```python
from build123d import *

# Parameters (mm, degrees)
ESQUISSE1_R                  = 1.15
ESQUISSE1_R_2                = 13.5
BOSS_EXTRU_1_DEPTH           = 8
ESQUISSE2_R                  = 13.5
ESQUISSE2_R_2                = 12.5
BOSS_EXTRU_2_DEPTH           = 2
ENL_V_MAT_EXTRU_1_DEPTH      = 3
R_P_TITION_CIRCULAIRE1_COUNT = 3
ESQUISSE4_W                  = 10
ESQUISSE4_H                  = 20
BOSS_EXTRU_3_DEPTH           = 40
PER_AGEAVANC_1_OUTLINE_R     = 2.25
PER_AGEAVANC_1_DEPTH         = 2.45
PER_AGEAVANC_1_DRAFT         = 45
PER_AGEAVANC_1_2_OUTLINE_R   = 2.25
PER_AGEAVANC_1_2_DEPTH       = 2.45
PER_AGEAVANC_1_2_DRAFT       = 45
ESQUISSE7_R                  = 2.25
ENL_V_MAT_EXTRU_2_DEPTH      = 66.754160325
CHANFREIN1_SIZE              = 1


# Read off the part's stored shape, not the designer's step: PerçageAvancé1
with BuildPart() as part:
    # Esquisse1 → Boss.-Extru.1 (new body)
    with BuildSketch(Plane(origin=(0, 0, 0), x_dir=(1, 0, 0), z_dir=(0, 1, 0))):
        with BuildLine():
            Line((20, -46.91), (20, 0))
            ThreePointArc((20, 0), (0, 20), (-20, 0))
            Line((-20, 0), (-20, -46.91))
            Line((-20, -46.91), (20, -46.91))
        make_face()
        with Locations(Location((0, 16.5, 0), (0, 0, 270))):
            Circle(ESQUISSE1_R, mode=Mode.SUBTRACT)
        with Locations(Location((-14.289419162, -8.25, 0), (0, 0, 270))):
            Circle(ESQUISSE1_R, mode=Mode.SUBTRACT)
        with Locations(Location((0, 0, 0), (0, 0, 270))):
            Circle(ESQUISSE1_R_2, mode=Mode.SUBTRACT)
        with Locations(Location((14.289419162, -8.25, 0), (0, 0, 270))):
            Circle(ESQUISSE1_R, mode=Mode.SUBTRACT)
    extrude(amount=BOSS_EXTRU_1_DEPTH)

    # Esquisse2 → Boss.-Extru.2 (add)
    with BuildSketch(Plane.XZ):
        with Locations(Location((0, 0, 0), (0, 0, 270))):
            Circle(ESQUISSE2_R)
        with Locations(Location((0, 0, 0), (0, 0, 270))):
            Circle(ESQUISSE2_R_2, mode=Mode.SUBTRACT)
    extrude(amount=-BOSS_EXTRU_2_DEPTH)

    # Esquisse3 → Enlèv. mat.-Extru.1 (cut)
    with BuildSketch(Plane.XZ):
        Polygon((-14.289419162, 5.882863896), (-12.239419162, 7.066431948), (-12.239419162, 9.433568052), (-14.289419162, 10.617136104), (-16.339419162, 9.433568052), (-16.339419162, 7.066431948), align=None)
    enl_v_mat_extru_1 = extrude(amount=-ENL_V_MAT_EXTRU_1_DEPTH, mode=Mode.SUBTRACT)

    # Répétition circulaire1: Enlèv. mat.-Extru.1 ×3 about axis
    r_p_tition_circulaire1_axis = Axis((0, 0, 0), (0, 1, 0))
    for i in range(1, R_P_TITION_CIRCULAIRE1_COUNT):
        add(enl_v_mat_extru_1.rotate(r_p_tition_circulaire1_axis, i * 360 / R_P_TITION_CIRCULAIRE1_COUNT), mode=Mode.SUBTRACT)

    # Esquisse4 → Boss.-Extru.3 (add)
    with BuildSketch(Plane.ZY.offset(20)):
        with Locations((41.91, 10)):
            Rectangle(ESQUISSE4_W, ESQUISSE4_H)
    extrude(amount=-BOSS_EXTRU_3_DEPTH)


with BuildPart() as per_ageavanc_1_tool:
    # PerçageAvancé1 outline → PerçageAvancé1 (with draft: the straight prism first)
    with BuildSketch(Plane.XY.offset(39.36)):
        with Locations((-12, 14)):
            Circle(PER_AGEAVANC_1_OUTLINE_R)
    extrude(amount=-PER_AGEAVANC_1_DEPTH)
    # PerçageAvancé1: the draft: its side faces are tilted about the plane it starts from
    per_ageavanc_1_sides = [per_ageavanc_1_tool.faces().sort_by_distance(p)[0] for p in [
        (-14.25, 14, 38.135),
    ]]
    draft(per_ageavanc_1_sides, Plane.XY.offset(39.36), PER_AGEAVANC_1_DRAFT)


with BuildPart() as part_1:
    add(part.part)

    # PerçageAvancé1: cut by per_ageavanc_1_tool
    add(per_ageavanc_1_tool.part, mode=Mode.SUBTRACT)


with BuildPart() as per_ageavanc_1_2_tool:
    # Per_ageAvanc_1 2 outline → Per_ageAvanc_1 2 (with draft: the straight prism first)
    with BuildSketch(Plane.XY.offset(39.36)):
        with Locations((12, 14)):
            Circle(PER_AGEAVANC_1_2_OUTLINE_R)
    extrude(amount=-PER_AGEAVANC_1_2_DEPTH)
    # Per_ageAvanc_1 2: the draft: its side faces are tilted about the plane it starts from
    per_ageavanc_1_2_sides = [per_ageavanc_1_2_tool.faces().sort_by_distance(p)[0] for p in [
        (9.75, 14, 38.135),
    ]]
    draft(per_ageavanc_1_2_sides, Plane.XY.offset(39.36), PER_AGEAVANC_1_2_DRAFT)


with BuildPart() as part_2:
    add(part_1.part)

    # Per_ageAvanc_1 2: cut by per_ageavanc_1_2_tool
    add(per_ageavanc_1_2_tool.part, mode=Mode.SUBTRACT)

    # Esquisse7 → Enlèv. mat.-Extru.2 (cut, through all)
    with BuildSketch(Plane(origin=(0, 0, 39.36), x_dir=(-1, 0, 0), z_dir=(0, 0, -1))):
        with Locations((-12, 14)):
            Circle(ESQUISSE7_R)
        with Locations((12, 14)):
            Circle(ESQUISSE7_R)
    extrude(amount=-ENL_V_MAT_EXTRU_2_DEPTH, mode=Mode.SUBTRACT)

    # Chanfrein1
    chanfrein1_edges = [part_2.edges().sort_by_distance(p)[0] for p in [
        (20, 8, 18.455),
        (20, 14, 36.91),
        (0, 20, 36.91),
        (-20, 14, 36.91),
        (-20, 8, 18.455),
        (0, 8, -20),
        (0, 0, -20),
        (0, 8, -13.5),
        (20, 0, 23.455),
        (-20, 0, 23.455),
    ]]
    chamfer(chanfrein1_edges, length=CHANFREIN1_SIZE)


solid = part_2.part
```
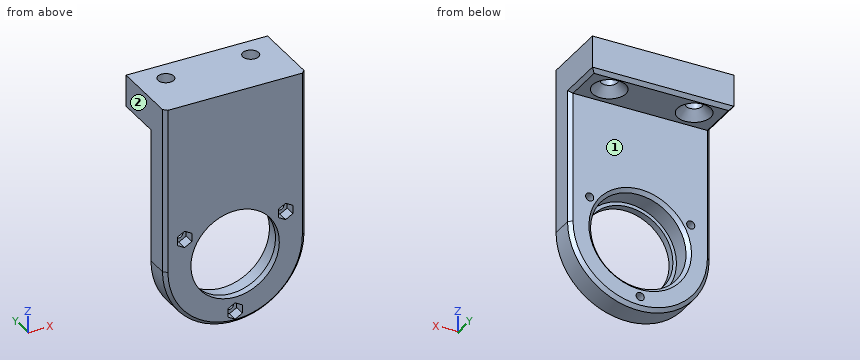
Could you check a few things on this model? Use its own coordinates, in mm. Face numbers are marked on the shaded views. A direction names the side the tool comes from. Round coordinates to 2 decimals unless told otherwise and drop trailing zeros. Loops run counter-clockwise (first coordinate to the right, second up) from the corner with the lowest first, then second, coordinate; pieces in that order, holes last. Notation, with made-up numbers: M 51,23.5 L 101,23.5 A21 cw 101,41.5 Z; hole C -39.75,28.25 d6. An arc over 180 degrees is marked long. Write item = value, one per line.
1. I want a section at A-A, the plane y = 5. Write out the boundary of the cut face in (x, z), and give its area (3 significant figures).
Results below:
outline = M -20,0 A20 ccw 20,0 L 20,46.91 L -20,46.91 Z; hole C -14.29,8.25 d2.3; hole C 0,0 d27; hole C 0,-16.5 d2.3; hole C 14.29,8.25 d2.3
area = 1,920 mm²
2. Will these pins go through, and if not, where does the flat tip stop? P1, Ø5.5, axis at x = -9.5, y = 14.5, coming from the -Z side; P2, Ø2, axis at x = -1, z = -17.5, coming from the -Y side; P3, Ø4, axis at y = 8, z = -11.5, coming from the +X side; P4, Ø21.5, axis at x = 0, z = 0, coming from the +Y side.
Results below:
P1 = 36.91
P2 = 0
P3 = 17.45
P4 = through
3. I need wall thicknesses on probe 1 along X at (y, z) = (14, 44); probe 2 along X at (y, z) = (5, 0); probe 3 along Y at (x, z) = (-12, 44). Which ranges of each line are inside material? Lowest first, please.
Results below:
probe_1 = -20 to -14.25, -9.75 to 9.75, 14.25 to 20
probe_2 = -20 to -13.5, 13.5 to 20
probe_3 = 0 to 11.75, 16.25 to 20
4. Which directions (+Z, -Z, +X, -X, +Y, -Y) give clear straight access to the entire face, cutting with the end or side of a thin tool? Please do the marked faces 1 and 2.
Results below:
face_1 = -Z, +X, -X, +Y
face_2 = +Z, -Z, -X, +Y, -Y
5. I want a section at C-C, the plane x = 11.5. Count the separate pieces of the cut face and the enclosed holes in it, and give its area (3 significant figures).
Results below:
separate_pieces = 3
enclosed_holes = 0
area = 468 mm²
6. I want a section at B-B, the plane y = 14. Write out the boundary of the cut face in (x, z), and give its area (3 significant figures).
Results below:
outline = M -20,37.91 L -19,36.91 L -16.7,36.91 L -14.25,39.36 L -14.25,46.91 L -20,46.91 Z; M -9.75,39.36 L -7.3,36.91 L 7.3,36.91 L 9.75,39.36 L 9.75,46.91 L -9.75,46.91 Z; M 14.25,39.36 L 16.7,36.91 L 19,36.91 L 20,37.91 L 20,46.91 L 14.25,46.91 Z
area = 297 mm²
